Build history of the part. All positions in model axes, mm. A direction names the side the tool comes from. Coordinates: 2 decimals unless noted, no trailing zeros. Order: outer loops, then holes, each group sorted by start corner. A loop starts at its lowest first (then second) coordinate and runs counter-clockwise, first axis right, second up. Notation, with made-up numbers: (11, 34.25) - (26, 34.25) arc R14 cw to (26, 55.25) - close; hole circle Ø5 at (-16.5, 37.5). An arc over 180 degrees is marked (long way). One line per item, written item: value.
from build123d import *

# Parameters (mm, degrees)
F3_W     = 15
F3_H     = 20
F3_W_2   = 55
F3_H_2   = 30
F4_DEPTH = 15
F5_R     = 15
F6_R     = 30
F7_R     = 14.99999
F9_DEPTH = 15.001


# Not quite as in the source:
# - a fillet or chamfer is up to 0.001 mm smaller than in the source, because OpenCascade refuses the exact size


with BuildPart() as f4:
    # F3 (on Front) → F4 (new body)
    with BuildSketch(Plane.XZ):
        with Locations((7.5, 10)):
            Rectangle(F3_W, F3_H)
        with Locations((-27.5, -15)):
            Rectangle(F3_W_2, F3_H_2)
        Polygon((15, 0), (0, 0), (0, -30), align=None)
    extrude(amount=F4_DEPTH)

    # F5
    f5_edges = [f4.edges().sort_by_distance(p)[0] for p in [
        (15, -7.5, 0),
    ]]
    fillet(f5_edges, radius=F5_R)

    # F6
    f6_edges = [f4.edges().sort_by_distance(p)[0] for p in [
        (0, -7.5, -30),
    ]]
    fillet(f6_edges, radius=F6_R)

    # F7 (radius 15 in the source; OpenCascade refuses exactly that, so slightly less here)
    f7_edges = [f4.edges().sort_by_distance(p)[0] for p in [
        (15, -7.5, 20),
    ]]
    fillet(f7_edges, radius=F7_R)

    # F8 (on face) → F9 (cut, through all)
    with BuildSketch(Plane(origin=(0, 0, 0), x_dir=(-1, 0, 0), z_dir=(0, 1, 0))):
        Polygon((25, 0), (55, -30), (55, 0), align=None)
    extrude(amount=-F9_DEPTH, mode=Mode.SUBTRACT)


solid = f4.part
1. 3-axis set-ups, long thin cutter, end or side, ignore diameter. For faces 1 (the face through (14.59, -7.6, 0.05)), 2 (the face through (-13, -7, 0)): which of +Z, -Z, +X, -X, +Y, -Y reach the whole face in a straight line?
Values found:
face 1: -Z, +X, +Y, -Y
face 2: +Z, -X, +Y, -Y
2. Band-saw the part on B-B, the plane x = -40. Give the cut face in (y, z), and give its area (3 significant figures).
Values found:
outline: (-15, -30) - (0, -30) - (0, -15) - (-15, -15) - close
area: 225 mm2
3. Probe line 1 along Z through (x, y) = (-19.5, -12); line 2 along Z through (x, y) = (-38.5, -13.75); line 3 along X through (y, z) = (-6, -22). List the from-to ranges inside material, lowest first.
Values found:
line 1: z = -30 to 0
line 2: z = -30 to -13.5
line 3: x = -47 to 1.86
4. Flat gauge pins, fed straight in: P1, Ø1.5, axis at x = -31, y = -2.5, coming from the +Z side; P2, Ø1, axis at y = -2, z = -18.5, coming from the -X side; P3, Ø4.5, axis at y = -4, z = 7.5, coming from the -X side. Where does each tip first touch, or does it go through?
Values found:
P1: stops at z = -5.25
P2: stops at x = -44
P3: stops at x = 0
5. Band-saw the part on C-C, the plane z = -7. Give the cut face in (x, y).
Values found:
outline: (-32, -15) - (11.5, -15) - (11.5, 0) - (-32, 0) - close
